Geometry check sheet. Reference: drawing and pictorial views, mm from the part's lowest x, y, z. A direction names the side the tool comes from. Round coordinates to 2 decimals unless told otherwise and drop trailing zeros. Write each loop counter-clockwise with the first axis right and the second up, starting at its lowest first coordinate (ties: lowest second). Pieces come first, ordered by that corner, then holes. Notation, with made-up numbers: (18, 72) -> (55, 72) arc R16 cw to (55, 99) -> close; hole circle Ø7 at (24, 85). An arc over 180 degrees is marked (long way). Answer as a JSON object with one key per item and string values. Group by question number.
(1) Scan lines: L1, parallel to Y at x = 1.25, z = 168; L2, parallel to Z at x = 10.75, y = 27. Record each from-to range of solid material in increasing order. Write a range as from..to.
(2) Sectioned sample at C-C on x = 12.75. Count the separate pieces of the cut face and the enclosed holes in it, and give its area (3 significant figures).
(3) Sectioned sample at B-B on z = 167. Record the cut outline in (x, y).
(4) Gauge pin test, flat ends, axial feed: pin 1 Ø5.5 at (x, z) = (10, 172) entering from -Y; pin 2 Ø6.5 at (x, y) = (13, 59) entering from +Z; pin 3 Ø5.5 at (x, z) = (9.5, 163.5) entering from +Y; pin 4 Ø5 at (y, z) = (55.5, 79.51) entering from +X. Record the tip position at first contact, or that the pin passes through.
(5) Set-up check for the marked faces 1 and 2: record each of +Z, -Z, +X, -X, +Y, -Y from which the full face is reachable in a straight line by a thin tool's end or side.
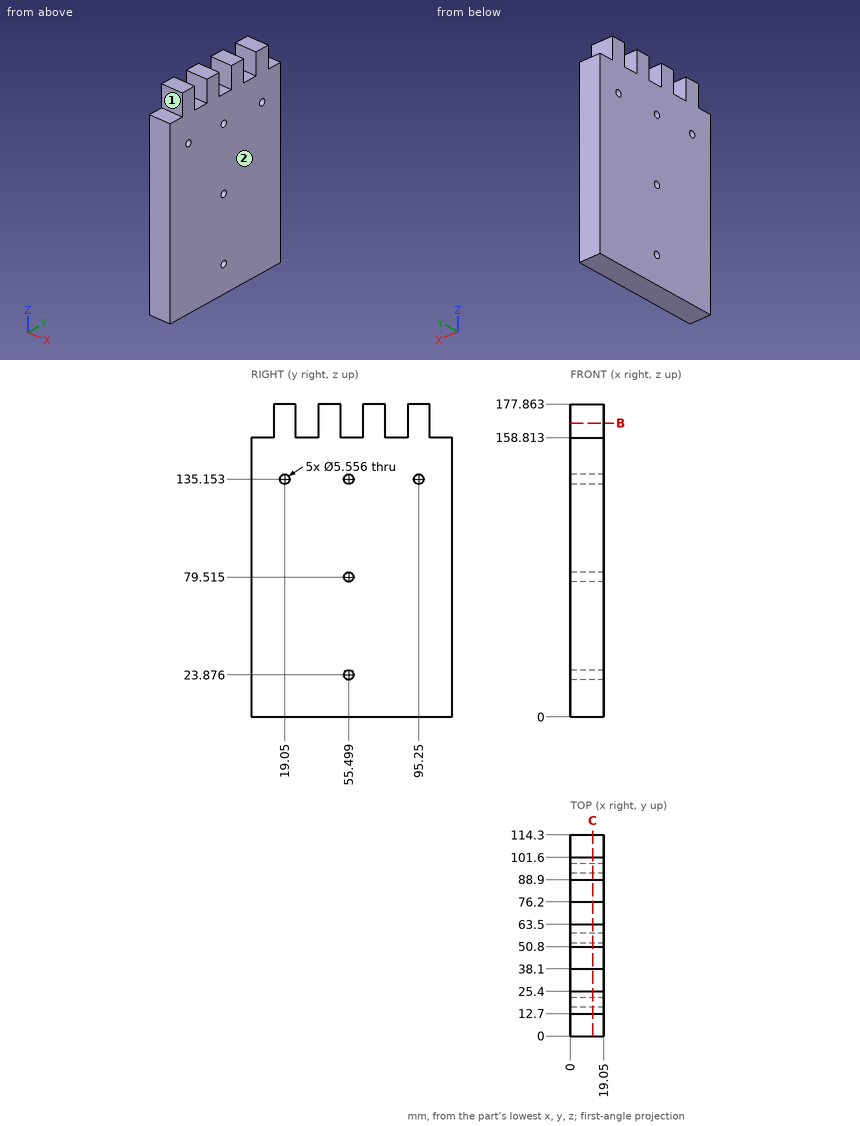
Computed values:
{
 "1": {"L1": "12.7..25.4, 38.1..50.8, 63.5..76.2, 88.9..101.6", "L2": "0..158.81"},
 "2": {"separate pieces": "1", "enclosed holes": "5", "area": "19,000 mm2"},
 "3": {"outline": "(0, 12.7) -> (19.05, 12.7) -> (19.05, 25.4) -> (0, 25.4) -> close; (0, 38.1) -> (19.05, 38.1) -> (19.05, 50.8) -> (0, 50.8) -> close; (0, 63.5) -> (19.05, 63.5) -> (19.05, 76.2) -> (0, 76.2) -> close; (0, 88.9) -> (19.05, 88.9) -> (19.05, 101.6) -> (0, 101.6) -> close"},
 "4": {"pin 1": "y = 12.7", "pin 2": "z = 158.81", "pin 3": "y = 101.6", "pin 4": "through"},
 "5": {"face 1": "+Z, +X, -X, -Y", "face 2": "+Z, -Z, +X, +Y, -Y"}
}
